Can you work these out from the model? Positions are in its coordinate system, mm. Face numbers are marked on the shaded views. Give positions to 0.01 mm unless a question says otherwise; leave off trailing zeros. Write each loop counter-clockwise with the first axis right and the second up, starting at its lowest first coordinate (ties: lowest second). Pieces come first, ordered by that corner, then holes. Notation, with made-up numbers: (-30.5, 45) -> (-10.5, 45) arc R33 ccw to (-10.5, 73) -> close; hole circle Ø8 at (37, -40). An arc over 180 degrees is marked (long way). Answer as CSV lines item,"result". Start each with the question number.
1. If we section it at C-C on z = 37.5: Write out the boundary of the cut face in (x, y).
2. If we section it at A-A on y = 0: Write out the boundary of the cut face in (x, z).
3. If we section it at D-D on y = -2.5: Write out the boundary of the cut face in (x, z).
4. I need wall thicknesses on line 1 (Z direction, x = 0, y = -0.5); line 2 (X direction, y = 0.5, z = 54); line 3 (X direction, y = 3, z = 14.5). Which ranges of each line are inside material? Lowest first, please. Write a range as [from, to].
5. I'm going to push a flat-ended pin straight in: P1, Ø1.2, axis at x = 0, y = 0, coming from the +Z side. Where does the tip first touch, or does it pass through?
6. If we section it at B-B on x = 0: Write out the boundary of the cut face in (y, z), plus the area to 3 significant figures.
7. If we mould it in two halves opening along Y, with no side actions, what happens to the marked faces 1, 2 and 3? For each: pulls with the +Y half, pulls with the -Y half, needs draft (parallel to the pull), parting line crosses it, or undercut.
```python
from build123d import *

# Parameters (mm, degrees)
BOSS_EXTRUDE1_DEPTH = 60
SKETCH2_W           = 1.5
SKETCH2_H           = 8
CUT_EXTRUDE1_DEPTH  = 10


with BuildPart() as part:
    # Sketch1 → Boss-Extrude1 (new body)
    with BuildSketch(Plane.XY):
        with BuildLine():
            Line((-2.645751311, -3), (2.645751311, -3))
            ThreePointArc((2.645751311, -3), (0, 4), (-2.645751311, -3))
        make_face()
    extrude(amount=BOSS_EXTRUDE1_DEPTH)

    # Sketch2 → Cut-Extrude1 (cut)
    with BuildSketch(Plane.XY.offset(60)):
        Rectangle(SKETCH2_W, SKETCH2_H)
    extrude(amount=-CUT_EXTRUDE1_DEPTH, mode=Mode.SUBTRACT)


solid = part.part
```
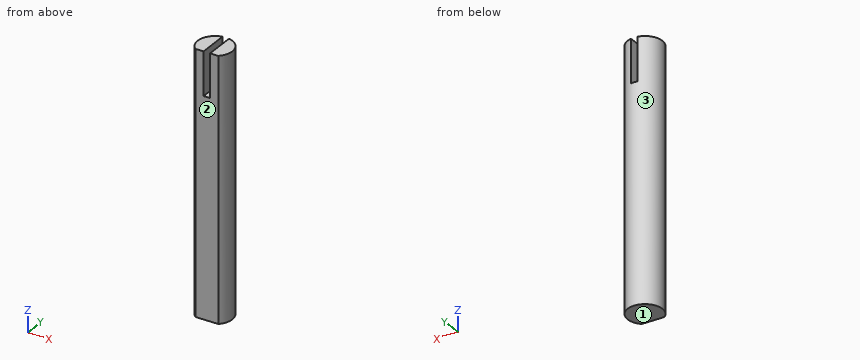
Computed values:
1,outline,"(-2.65, -3) -> (2.65, -3) arc R4 ccw (long way) to start"
2,outline,"(-4, 0) -> (4, 0) -> (4, 60) -> (0.75, 60) -> (0.75, 50) -> (-0.75, 50) -> (-0.75, 60) -> (-4, 60) -> close"
3,outline,"(-3.12, 0) -> (3.12, 0) -> (3.12, 60) -> (0.75, 60) -> (0.75, 50) -> (-0.75, 50) -> (-0.75, 60) -> (-3.12, 60) -> close"
4,line 1,"z = [0, 50]"
4,line 2,"x = [-3.97, -0.75], [0.75, 3.97]"
4,line 3,"x = [-2.65, 2.65]"
5,P1,"stops at z = 50"
6,outline,"(-3, 0) -> (4, 0) -> (4, 50) -> (-3, 50) -> close"
6,area,"350 mm2"
7,face 1,"needs draft"
7,face 2,"pulls with the -Y half"
7,face 3,"parting line crosses it"
